Can you work these out from the drawing? Everything is in mm from the part's minimum corner. Round coordinates to 2 decimals unless told otherwise and drop trailing zeros. Loops run counter-clockwise (first coordinate to the right, second up) from the corner with the lowest first, then second, coordinate; pieces in that order, holes last. Notation, with made-up numbers: (-31, 7) -> (13, 7) arc R14 ccw to (13, 13) -> close; hole circle Ø7 at (-32.5, 57.25). An arc over 180 degrees is marked (long way). One line per item, written item: value.
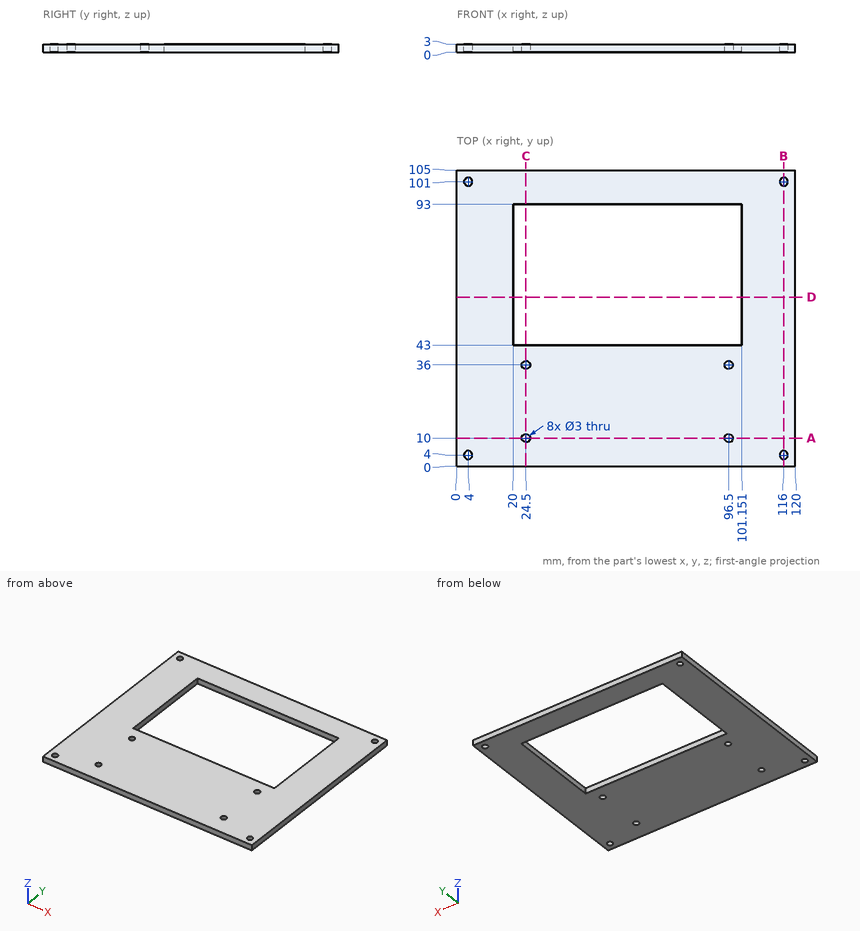
(1) For pin 1 Ø1.8 at (x, y) = (4, 4) entering from +Z, with a flat end and sliding along its axis, tell me the tip position at first contact or that it passes through.
Results below:
pin 1: passes through
(2) Imagine slicing it at C-C on x = 24.5. Write out the boundary of the cut face in (y, z).
Results below:
outline: (0, 0) -> (8.5, 0) -> (8.5, 3) -> (0, 3) -> close; (11.5, 0) -> (34.5, 0) -> (34.5, 3) -> (11.5, 3) -> close; (37.5, 0) -> (43, 0) -> (43, 3) -> (37.5, 3) -> close; (93, 0) -> (105, 0) -> (105, 3) -> (93, 3) -> close
(3) Please list where these lines run through material, in increasing order: L1, parallel to Y at x = 24.5, z = 0.6; L2, parallel to X at y = 101, z = 0.8; L3, parallel to Y at x = 116, z = 2.35.
Results below:
L1: y = 0 to 8.5, 11.5 to 34.5, 37.5 to 43, 93 to 105
L2: x = 0 to 2.5, 5.5 to 114.5, 117.5 to 120
L3: y = 0 to 2.5, 5.5 to 99.5, 102.5 to 105
(4) Imagine slicing it at A-A on y = 10. Write out the boundary of the cut face in (x, z), then the cut area to 3 significant figures.
Results below:
outline: (0, 0) -> (23, 0) -> (23, 3) -> (0, 3) -> close; (26, 0) -> (95, 0) -> (95, 3) -> (26, 3) -> close; (98, 0) -> (120, 0) -> (120, 3) -> (98, 3) -> close
area: 342 mm²
(5) Imagine slicing it at D-D on y = 60. Write out the boundary of the cut face in (x, z).
Results below:
outline: (0, 0) -> (20, 0) -> (20, 3) -> (0, 3) -> close; (101.15, 0) -> (120, 0) -> (120, 3) -> (101.15, 3) -> close
(6) Imagine slicing it at B-B on x = 116. Write out the boundary of the cut face in (y, z), then the cut area to 3 significant figures.
Results below:
outline: (0, 0) -> (2.5, 0) -> (2.5, 3) -> (0, 3) -> close; (5.5, 0) -> (99.5, 0) -> (99.5, 3) -> (5.5, 3) -> close; (102.5, 0) -> (105, 0) -> (105, 3) -> (102.5, 3) -> close
area: 297 mm²
